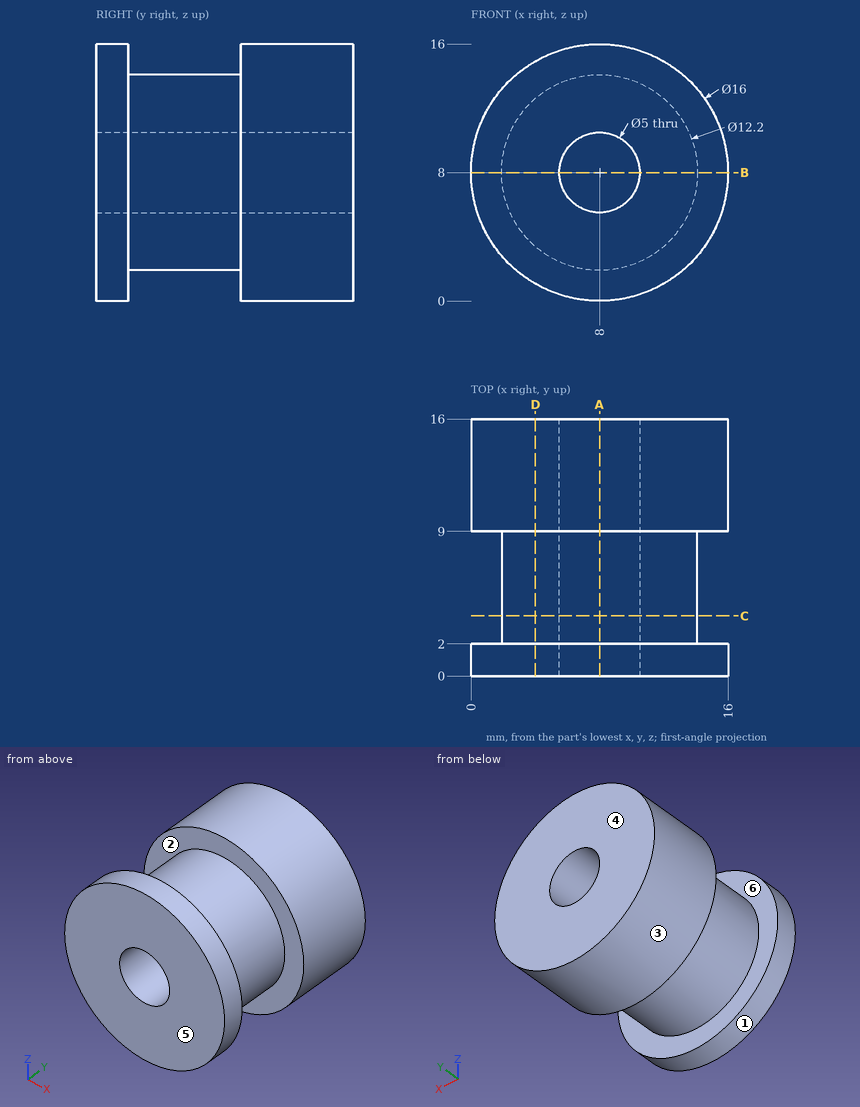
Input: dimensioned drawing with shaded views. Units: mm. Origin: part minimum x, y, z. A direction names the side the tool comes from. Coordinates: 2 decimals unless noted, no trailing zeros. Order: outer loops, then holes, each group sorted by start corner. A loop starts at its lowest first (then second) coordinate and runs counter-clockwise, first axis right, second up.
1. Cut plane A-A, the plane x = 8. Return loops of the section in (y, z), plus the area to 3 significant figures.
Checked values:
outline: (0, 0) - (2, 0) - (2, 1.9) - (9, 1.9) - (9, 0) - (16, 0) - (16, 5.5) - (0, 5.5) - close; (0, 10.5) - (16, 10.5) - (16, 16) - (9, 16) - (9, 14.1) - (2, 14.1) - (2, 16) - (0, 16) - close
area: 149 mm2
2. Access query for the marked faces 1 and 2. Directions: +Z, -Z, +X, -X, +Y, -Y. A direction counts if a zero-diameter tool reaches every point of the face in a straight line with its end or side. Return the directions, or none.
Checked values:
face 1: +Y, -Y
face 2: none
3. Cut plane B-B, the plane z = 8. Return loops of the section in (x, y).
Checked values:
outline: (0, 0) - (5.5, 0) - (5.5, 16) - (0, 16) - (0, 9) - (1.9, 9) - (1.9, 2) - (0, 2) - close; (10.5, 0) - (16, 0) - (16, 2) - (14.1, 2) - (14.1, 9) - (16, 9) - (16, 16) - (10.5, 16) - close
4. Cut plane D-D, the plane x = 4. Return loops of the section in (y, z), plus the area to 3 significant figures.
Checked values:
outline: (0, 1.07) - (2, 1.07) - (2, 3.39) - (9, 3.39) - (9, 1.07) - (16, 1.07) - (16, 14.93) - (9, 14.93) - (9, 12.61) - (2, 12.61) - (2, 14.93) - (0, 14.93) - close
area: 189 mm2
5. Draft query along Y for the marked faces 3, 4, 5 and 6. Return one class per face: +Y half, -Y half, draft (parallel to the pull), parting line (faces both ways), or undercut.
Checked values:
face 3: draft
face 4: +Y half
face 5: -Y half
face 6: undercut
6. Ray query, line 1 along Z through (x, y) = (8, 8.5); line 2 along Y through (x, z) = (1.5, 3.75). Return the intervals inside material, ascending.
Checked values:
line 1: z = 1.9 to 5.5, 10.5 to 14.1
line 2: y = 0 to 2, 9 to 16
7. Cut plane C-C, the plane y = 3.75. Return loops of the section in (x, z), plus the area to 3 significant figures.
Checked values:
outline: circle Ø12.2 at (8, 8); hole circle Ø5 at (8, 8)
area: 97.3 mm2
8. Contact query for flat-ended pins moving along their axis: P1, Ø8, axis at x = 7, y = 4.5, coming from the +Z side; P2, Ø2, axis at x = 2, y = 13, coming from the -Z side (3 decimals); P3, Ø8, axis at x = 2, y = 5.5, coming from the +Z side. Output: stop coordinate, or through.
Checked values:
P1: stops at z = 16
P2: stops at z = 1.755
P3: stops at z = 14.89
